Autodesk Inventor part; units mm, degrees
ref_plane "YZ Plane" through (0, 0, 0) normal (1, 0, 0) x (0, 1, 0)
ref_plane "XZ Plane" through (0, 0, 0) normal (0, 1, 0) x (-1, 0, 0)
ref_plane "XY Plane" through (0, 0, 0) normal (0, 0, 1) x (1, 0, 0)
sketch "スケッチ1" plane through (0, 0, 0) normal (0, 0, 1) x (1, 0, 0)
  line L0 (0, 0) -> (-90.3, 0)
  line L1 (-90.3, 0) -> (-90.3, 64.35)
  line L2 (-90.3, 64.35) -> (0, 64.35)
  line L3 (0, 64.35) -> (0, 0)
  line L4 (-90.3, 21.15) -> (0, 21.15)
  line L5 (-55.219, 21.15) -> (-37.813, 0)
  line L6 (-90.3, 29.15) -> (0, 29.15)
  line L7 (-80.3, 29.15) -> (-67.1, 29.15)
  line L8 (-67.1, 29.15) -> (-67.1, 34.35)
  line L9 (-67.1, 34.35) -> (-80.3, 34.35)
  line L10 (-80.3, 34.35) -> (-80.3, 29.15)
  line L11 (-67.1, 29.15) -> (-67.1, 21.15)
  line L12 (-38.44, 64.35) -> (0, 54.9793)
  dimension "d0" = 90.3
  dimension "d1" = 64.35
  dimension "d2" = 21.15
  dimension "d3" = 55.219
  dimension "d4" = 37.813
  dimension "d5" = 35.2
  dimension "d6" = 10
  dimension "d7" = 5.2
  dimension "d8" = 13.2
  dimension "d9" = 166.3
  dimension "d10" = 51.86
extrude "押し出し1" add sketch "スケッチ1" along normal blind 3 contours L0 L5 L4 L3 | L4 L11 L6 L3 | L6 L8 L9 L10 L1 L2 L12 L3
sketch "スケッチ2" plane through (0, 0, 3) normal (0, 0, 1) x (1, 0, 0)
  line L0 (-85.1, 34.75) -> (-53.1, 34.75)
  line L1 (-53.1, 34.75) -> (-53.1, 50.75)
  line L2 (-53.1, 50.75) -> (-85.1, 50.75)
  line L3 (-85.1, 50.75) -> (-85.1, 34.75)
  line L4 (-90.3, 29.15) -> (-80.3, 29.15)
  line L5 (-90.3, 64.35) -> (-90.3, 29.15)
  line L6 (-8.4, 4.75) -> (-24.4, 4.75)
  line L7 (-24.4, 4.75) -> (-24.4, 36.75)
  line L8 (-24.4, 36.75) -> (-8.4, 36.75)
  line L9 (-8.4, 36.75) -> (-8.4, 4.75)
  line L10 (0, 0) -> (0, 54.9793)
  line L11 (-37.813, 0) -> (0, 0)
  dimension "d13" = 5.6
  dimension "d14" = 5.2
  dimension "d15" = 16
  dimension "d16" = 32
  dimension "d17" = 8.4
  dimension "d18" = 4.75
  dimension "d19" = 16
  dimension "d20" = 32
hole "穴1" at (-85.1, 50.75, 3) at (-85.1, 34.75, 3) at (-53.1, 34.75, 3) at (-53.1, 50.75, 3) at (-24.4, 4.75, 3) at (-8.4, 4.75, 3) at (-8.4, 36.75, 3) at (-24.4, 36.75, 3) direction (0, 0, -1) diameter 2.5 end through all
fillet "フィレット1" radius 1 11 edges at (0, 0, 1.5) (0, 54.9793, 1.5) (-90.3, 64.35, 1.5) (-90.3, 29.15, 1.5) (-80.3, 29.15, 1.5) (-80.3, 34.35, 1.5) (-67.1, 34.35, 1.5) (-67.1, 21.15, 1.5) (-55.219, 21.15, 1.5) (-37.813, 0, 1.5) (-38.44, 64.35, 1.5)
sketch "スケッチ3" plane through (0, 0, 0) normal (0, 0, -1) x (-1, 0, 0)
  line L0 (31.65, 18.75) -> (39.65, 18.75)
  line L1 (39.65, 18.75) -> (39.65, 32.75)
  line L2 (39.65, 32.75) -> (31.65, 32.75)
  line L3 (31.65, 32.75) -> (31.65, 18.75)
  circle A0 centre (24.4, 4.75) radius 1.25
  circle A1 centre (24.4, 36.75) radius 1.25
  point P0 (0, 0)
  dimension "d29" = 14
  dimension "d30" = 14
  dimension "d31" = 8
  dimension "d32" = 6
extrude "押し出し2" cut sketch "スケッチ3" against normal blind 10 contours L3 L2 L1 L0
fillet "フィレット2" radius 1 4 edges at (-31.65, 18.75, 1.5) (-31.65, 32.75, 1.5) (-39.65, 32.75, 1.5) (-39.65, 18.75, 1.5)
equation "\"BendRadius\" = Thickness"
equation "\"BendReliefWidth\" = Thickness"
equation "\"BendReliefDepth\" = 0.5 * Thickness"
equation "\"CornerReliefSize\" = 4 * Thickness"
equation "\"MinimumRemnant\" = 2 * Thickness"
equation "\"TransitionRadius\" = BendRadius"
equation "\"JacobiRadiusSize\" = BendRadius"
equation "\"GapSize\" = Thickness"
properties part number "connectplate1" material "アルミニウム 6061"
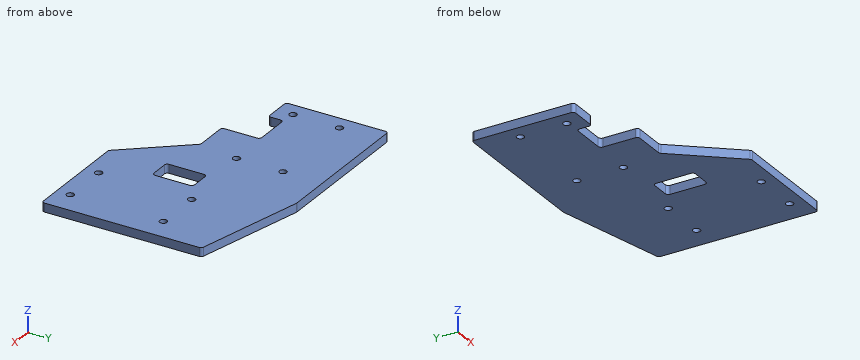
Geometry check sheet. Reference: the model listing, model coordinates, mm. Give positions to 0.01 mm unless a question says otherwise; leave off trailing zeros. Loops run counter-clockwise (first coordinate to the right, second up) from the corner with the lowest first, then second, coordinate; pieces in that order, holes last. Notation, with made-up numbers: M 74,84.5 L 90,84.5 A19 cw 90,93.5 Z; hole C 75,2.25 d2. An arc over 180 degrees is marked long. Write each question's results on one line, items separated by ' | '.
1) Section check A-A, the plane y = 50.75. Record the boundary of the cut face in (x, z), plus the area to 3 significant figures.
Answers follow:
outline: M -90.3,0 L -86.35,0 L -86.35,3 L -90.3,3 Z; M -83.85,0 L -54.35,0 L -54.35,3 L -83.85,3 Z; M -51.85,0 L 0,0 L 0,3 L -51.85,3 Z | area: 256 mm2
2) Section check B-B, the plane x = -85.1. Record the boundary of the cut face in (y, z), plus the area to 3 significant figures.
Answers follow:
outline: M 29.15,0 L 33.5,0 L 33.5,3 L 29.15,3 Z; M 36,0 L 49.5,0 L 49.5,3 L 36,3 Z; M 52,0 L 64.35,0 L 64.35,3 L 52,3 Z | area: 90.6 mm2
3) Section check C-C, the plane y = 26.5. Record the boundary of the cut face in (x, z), plus the area to 3 significant figures.
Answers follow:
outline: M -67.1,0 L -39.65,0 L -39.65,3 L -67.1,3 Z; M -31.65,0 L 0,0 L 0,3 L -31.65,3 Z | area: 177 mm2
4) Thickness scan on line 1 (X direction, y = 36.75, z = 0.8); line 2 (X direction, y = 50.75, z = 1.45); line 3 (Y direction, x = -8.4, z = 2.25). Record the ranges inside material, lowest first.
Answers follow:
line 1: -90.3 to -25.65, -23.15 to -9.65, -7.15 to 0 | line 2: -90.3 to -86.35, -83.85 to -54.35, -51.85 to 0 | line 3: 0 to 3.5, 6 to 35.5, 38 to 57.03
5) Gauge pin test, flat ends, axial feed: pin 1 (0.9 mm diameter, centred on x = -34.5, z = 1.5, fed in from +Y); pin 2 (1.5 mm diameter, centred on x = -63.5, z = 1.5, fed in from -Y); pin 3 (0.9 mm diameter, centred on y = 24.5, z = 1, fed in from -X). Record the tip position at first contact, or that the pin passes through.
Answers follow:
pin 1: y = 63.5 | pin 2: y = 21.15 | pin 3: x = -67.1
6) Section check D-D, the plane z = 1.7. Count the separate pieces of the cut face and the enclosed holes in it, plus the area to 3 significant figures.
Answers follow:
separate pieces: 1 | enclosed holes: 9 | area: 4,300 mm2
